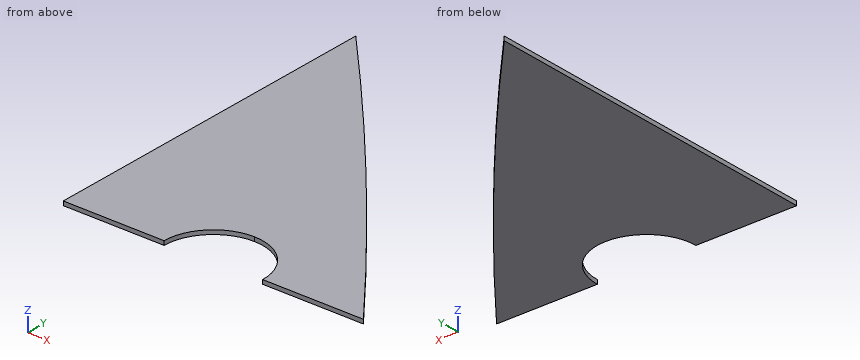
```python
from build123d import *

# Parameters (mm, degrees)
F1_DEPTH = 25.4


with BuildPart() as f1:
    # F0 (on Top) → F1 (new body)
    with BuildSketch(Plane.XY):
        with BuildLine():
            Line((-963.168343, 4128.799945), (-963.168343, 1967.513945))
            Line((-963.168343, 1967.513945), (-340.868343, 1967.513945))
            ThreePointArc((-340.868343, 1967.513945), (-251.59449, 2183.040092), (-36.068343, 2272.313945))
            Line((-36.068343, 2272.313945), (-36.068343, 3096.035945))
            ThreePointArc((-36.068343, 3096.035945), (-494.106465, 3617.365893), (-963.168343, 4128.799945))
        make_face()
        with BuildLine():
            Line((-36.068343, 3096.035945), (-36.068343, 2272.313945))
            ThreePointArc((-36.068343, 2272.313945), (179.457803, 2183.040092), (268.731657, 1967.513945))
            Line((268.731657, 1967.513945), (891.031657, 1967.513945))
            ThreePointArc((891.031657, 1967.513945), (433.820002, 2536.982003), (-36.068343, 3096.035945))
        make_face()
    extrude(amount=F1_DEPTH)


solid = f1.part
```
Model file for the job. Use its own axes, mm. Coordinates: 2 decimals unless noted, no trailing zeros. Loops run counter-clockwise (first coordinate to the right, second up) from the corner with the lowest first, then second, coordinate; pieces in that order, holes last. Notation, with made-up numbers: (83, 43) - (138, 43) arc R15 ccw to (138, 59) - close; hole circle Ø11 at (-34.75, -29). An arc over 180 degrees is marked (long way). Write item = value, one per line. Start each with the question number.
Item 1: Saw through at B-B, the plane y = 3917. List the corners of the cut face in (x, z), then the cut area to 3 significant figures.
Item 2: Drop flat-ended pins along their axis: pin 1 Ø4 at (x, z) = (-692, 3.5) entering from +Y; pin 2 Ø2 at (y, z) = (3693.5, 19) entering from +X; pin 3 Ø2 at (x, z) = (72.5, 17.5) entering from -Y. Give the stop position or say it passes through.
Item 3: Saw through at C-C, the plane x = -735. List the corners of the cut face in (y, z), then the cut area to 3 significant figures.
Item 4: Wall check: probe 1 along X at (y, z) = (2067.5, 12); probe 2 along Y at (x, z) = (-823, 5.5); probe 3 along X at (y, z) = (2214, 21.75). Give the ranges that are in metal, low to high. Write a range as [from, to].
Item 5: Saw through at A-A, the plane z = 14. List the corners of the cut face in (x, y), then the cut area to 3 significant figures.
Answers:
q1.outline = (-963.17, 0) - (-766.47, 0) - (-766.47, 25.4) - (-963.17, 25.4) - close
q1.area = 5,000 mm2
q2.pin_1 = 3838
q2.pin_2 = -561.76
q2.pin_3 = 2251.94
q3.outline = (1967.51, 0) - (3882.76, 0) - (3882.76, 25.4) - (1967.51, 25.4) - close
q3.area = 48,600 mm2
q4.probe_1 = [-963.17, -324], [251.87, 812.27]
q4.probe_2 = [1967.51, 3978.26]
q4.probe_3 = [-963.17, -215.37], [143.23, 695.71]
q5.outline = (-963.17, 1967.51) - (-340.87, 1967.51) arc R304.8 cw to (-36.07, 2272.31) arc R304.8 cw to (268.73, 1967.51) - (891.03, 1967.51) arc R32508.89 ccw to (-36.07, 3096.04) arc R32508.89 ccw to (-963.17, 4128.8) - close
q5.area = 1,920,000 mm2
